```python
from build123d import *

# Parameters (mm, degrees)
BOSS_EXTRUDE1_DEPTH = 3
FILLET1_R           = 1


with BuildPart() as part:
    # Sketch1 → Boss-Extrude1 (new body)
    with BuildSketch(Plane(origin=(0, 0, 0), x_dir=(1, 0, 0), z_dir=(0, 1, 0))):
        with BuildLine():
            ThreePointArc((8.15, 0), (7.036423097, 4.112329024), (4, 7.100880227))
            Line((4, 7.100880227), (4, 1.105667219))
            ThreePointArc((4, 1.105667219), (4.112329024, 0.55789784), (4.15, 0))
            ThreePointArc((4.15, 0), (-0.55789784, -4.112329024), (-4, 1.105667219))
            Line((-4, 1.105667219), (-4, 7.100880227))
            ThreePointArc((-4, 7.100880227), (-4.112329024, -7.036423097), (8.15, 0))
        make_face()
    extrude(amount=BOSS_EXTRUDE1_DEPTH)

    # Fillet1
    fillet1_edges = [part.edges().sort_by_distance(p)[0] for p in [
        (4, 1.5, -7.100880227),
        (-4, 1.5, -7.100880227),
    ]]
    fillet(fillet1_edges, radius=FILLET1_R)


solid = part.part
```
The listing builds one solid part. Answer for the finished solid, in the listing's coordinates (mm). A direction names the side the tool comes from. Give positions to 0.01 mm unless a question says otherwise; leave off trailing zeros. Write each loop counter-clockwise with the first axis right and the second up, starting at its lowest first coordinate (ties: lowest second). Pieces come first, ordered by that corner, then holes. Notation, with made-up numbers: (69.25, 62.25) -> (83.25, 62.25) arc R32 cw to (83.25, 95.25) -> close; hole circle Ø10 at (2, 28). An arc over 180 degrees is marked (long way). Write item = value, one per line. Start each with the question number.
1) The part is cut by section D-D, the plane x = 0. Determine the outline of the cut face in (y, z).
2) The part is cut by section B-B, the plane y = 2.2. Determine the outline of the cut face in (x, z), and give its area (3 significant figures).
3) Determine the mould class of faces 3 (the face through (-4, 1, -3)), 4 (the face through (2, 3, 4)) for opening direction X: +X half, -X half, draft (parallel to the pull), parting line (faces both ways), or undercut.
4) Which of the six approach directions +Z, -Z, +X, -X, +Y, -Y give full straight-line access (tool end or side, diameter ignored) to faces 1 (the face through (4, 1, -3)), 2 (the face through (2, 0, 4))?
5) Each of these flat-tipped pins is pushed along its axis until it touches: pin 1 (1 mm diameter, centred on x = -6.5, y = 2.5, fed in from +Z); pin 2 (1.5 mm diameter, centred on y = 1, z = -2.5, fed in from +X). Where does it stop, or does it pass through?
6) The part is cut by section A-A, the plane z = 3.5. Determine the outline of the cut face in (x, y), and give its area (3 significant figures).
7) The part is cut by section C-C, the plane z = -1.5. Determine the outline of the cut face in (x, y).
8) Straight lines are drawn through the part: line 1 along Z through (x, y) = (0, 1.5); line 2 along X through (y, z) = (2, 3.5); line 3 along X through (y, z) = (0.35, 2.75). For each, find the intervals that lie inside material, in ascending order.
Solutions:
q1.outline = (0, 4.15) -> (3, 4.15) -> (3, 8.15) -> (0, 8.15) -> close
q2.outline = (-5.7, -5.83) arc R1 ccw to (-4, -5.11) -> (-4, -1.11) arc R4.15 cw (long way) to (4, -1.11) -> (4, -5.11) arc R1 ccw to (5.7, -5.83) arc R8.15 ccw (long way) to start
q2.area = 117 mm²
q3.face_3 = undercut
q3.face_4 = draft
q4.face_1 = -Z, +Y, -Y
q4.face_2 = +Z, -Z, +X, -X, -Y
q5.pin_1 = 5.52
q5.pin_2 = 7.96
q6.outline = (-7.36, 0) -> (-2.23, 0) -> (-2.23, 3) -> (-7.36, 3) -> close; (2.23, 0) -> (7.36, 0) -> (7.36, 3) -> (2.23, 3) -> close
q6.area = 30.8 mm²
q7.outline = (-8.01, 0) -> (-4, 0) -> (-4, 3) -> (-8.01, 3) -> close; (4, 0) -> (8.01, 0) -> (8.01, 3) -> (4, 3) -> close
q8.line_1 = 4.15 to 8.15
q8.line_2 = -7.36 to -2.23, 2.23 to 7.36
q8.line_3 = -7.67 to -3.11, 3.11 to 7.67
